```python
from build123d import *

# Parameters (mm, degrees)
CYLINDER003_R          = 4
CYLINDER003_DEPTH      = 5
CYLINDER002_R          = 4
CYLINDER002_DEPTH      = 5
CYLINDER001_R          = 4
CYLINDER001_DEPTH      = 5
CYLINDER_R             = 4
CYLINDER_DEPTH         = 5
CONE003_ROLL_ANGLE     = 90
CONE002_ROLL_ANGLE     = 90
CONE001_ROLL_ANGLE     = -90
CONE_ROLL_ANGLE        = -90
BOX001_W               = 60
BOX001_H               = 20
BOX001_DEPTH           = 50
SKETCH001_W            = 57
SKETCH001_H            = 16.7
POCKET001_DEPTH        = 50
PAD_DEPTH              = 6
BOX_W                  = 120
BOX_H                  = 20
BOX_DEPTH              = 3
SKETCH_R               = 1.75
POCKET_DEPTH           = 3.001
CHAMFER_SIZE           = 3
CHAMFER001_SIZE        = 2
FILLET_R               = 1
FILLET_PLACEMENT_ANGLE = 90


with BuildPart() as cylinder003:
    # Cylinder003 → Cylinder003 (new body)
    with BuildSketch(Plane(origin=(50, 7, 3), x_dir=(1, 0, 0), z_dir=(0, 0, 1))):
        Circle(CYLINDER003_R)
    extrude(amount=CYLINDER003_DEPTH)


with BuildPart() as cylinder002:
    # Cylinder002 → Cylinder002 (new body)
    with BuildSketch(Plane(origin=(30, 7, 3), x_dir=(1, 0, 0), z_dir=(0, 0, 1))):
        Circle(CYLINDER002_R)
    extrude(amount=CYLINDER002_DEPTH)


with BuildPart() as cylinder001:
    # Cylinder001 → Cylinder001 (new body)
    with BuildSketch(Plane(origin=(50, -7, 3), x_dir=(1, 0, 0), z_dir=(0, 0, 1))):
        Circle(CYLINDER001_R)
    extrude(amount=CYLINDER001_DEPTH)


with BuildPart() as cylinder:
    # Cylinder → Cylinder (new body)
    with BuildSketch(Plane(origin=(30, -7, 3), x_dir=(1, 0, 0), z_dir=(0, 0, 1))):
        Circle(CYLINDER_R)
    extrude(amount=CYLINDER_DEPTH)


with BuildPart() as cone003:
    # Cone003 → Cone003 (revolve)
    with BuildSketch(Plane.XZ):
        Polygon((0, 0), (3, 0), (1.75, 3), (0, 3), align=None)
    revolve(axis=Axis((0, 0, 0), (0, 0, 1)))


with BuildPart() as cone003_1:
    # Cone003 roll: moved
    add(cone003.part.rotate(Axis((0, 0, 0), (1, 0, 0)), CONE003_ROLL_ANGLE))


with BuildPart() as cone003_2:
    # Cone003 placement: moved
    add(cone003_1.part.moved(Location((75, 10, 43))))


with BuildPart() as cone002:
    # Cone002 → Cone002 (revolve)
    with BuildSketch(Plane.XZ):
        Polygon((0, 0), (3, 0), (1.75, 3), (0, 3), align=None)
    revolve(axis=Axis((0, 0, 0), (0, 0, 1)))


with BuildPart() as cone002_1:
    # Cone002 roll: moved
    add(cone002.part.rotate(Axis((0, 0, 0), (1, 0, 0)), CONE002_ROLL_ANGLE))


with BuildPart() as cone002_2:
    # Cone002 placement: moved
    add(cone002_1.part.moved(Location((105, 10, 13))))


with BuildPart() as cone001:
    # Cone001 → Cone001 (revolve)
    with BuildSketch(Plane.XZ):
        Polygon((0, 0), (3, 0), (1.75, 3), (0, 3), align=None)
    revolve(axis=Axis((0, 0, 0), (0, 0, 1)))


with BuildPart() as cone001_1:
    # Cone001 roll: moved
    add(cone001.part.rotate(Axis((0, 0, 0), (1, 0, 0)), CONE001_ROLL_ANGLE))


with BuildPart() as cone001_2:
    # Cone001 placement: moved
    add(cone001_1.part.moved(Location((105, -10, 43))))


with BuildPart() as cone:
    # Cone → Cone (revolve)
    with BuildSketch(Plane.XZ):
        Polygon((0, 0), (3, 0), (1.75, 3), (0, 3), align=None)
    revolve(axis=Axis((0, 0, 0), (0, 0, 1)))


with BuildPart() as cone_1:
    # Cone roll: moved
    add(cone.part.rotate(Axis((0, 0, 0), (1, 0, 0)), CONE_ROLL_ANGLE))


with BuildPart() as cone_2:
    # Cone placement: moved
    add(cone_1.part.moved(Location((75, -10, 13))))


with BuildPart() as obj1:
    # Box001 → Box001 (new body)
    with BuildSketch(Plane(origin=(60, -10, 3), x_dir=(1, 0, 0), z_dir=(0, 0, 1))):
        with Locations((30, 10)):
            Rectangle(BOX001_W, BOX001_H)
    extrude(amount=BOX001_DEPTH)

    # Sketch001 → Pocket001 (cut)
    with BuildSketch(Plane(origin=(60, -10, 53), x_dir=(1, 0, 0), z_dir=(0, 0, 1))):
        with Locations((31.5, 10)):
            Rectangle(SKETCH001_W, SKETCH001_H)
    extrude(amount=-POCKET001_DEPTH, mode=Mode.SUBTRACT)

    # Cut: cut Cone
    add(cone_2.part, mode=Mode.SUBTRACT)

    # Cut001: cut Cone001
    add(cone001_2.part, mode=Mode.SUBTRACT)

    # Cut002: cut Cone002
    add(cone002_2.part, mode=Mode.SUBTRACT)

    # Cut003: cut Cone003
    add(cone003_2.part, mode=Mode.SUBTRACT)


with BuildPart() as triangle:
    # Sketch002 → Pad (new body)
    with BuildSketch(Plane.XZ.offset(-3)):
        Polygon((0, 3), (60, 53), (60, 3), align=None)
    extrude(amount=PAD_DEPTH)


with BuildPart() as triangle_y:
    # Box → Box (new body)
    with BuildSketch(Plane(origin=(0, -10, 0), x_dir=(1, 0, 0), z_dir=(0, 0, 1))):
        with Locations((60, 10)):
            Rectangle(BOX_W, BOX_H)
    extrude(amount=BOX_DEPTH)

    # Sketch → Pocket (cut, through all)
    with BuildSketch(Plane(origin=(0, -10, 3), x_dir=(1, 0, 0), z_dir=(0, 0, 1))):
        with Locations((30, 17)):
            Circle(SKETCH_R)
        with Locations((30, 3)):
            Circle(SKETCH_R)
        with Locations((50, 17)):
            Circle(SKETCH_R)
        with Locations((50, 3)):
            Circle(SKETCH_R)
    extrude(amount=-POCKET_DEPTH, mode=Mode.SUBTRACT)

    # Fusion: union obj1, triangle
    add(obj1.part)
    add(triangle.part)

    # Chamfer
    chamfer_edges = [triangle_y.edges().sort_by_distance(p)[0] for p in [
        (60, -3, 28),
        (60, 3, 28),
    ]]
    chamfer(chamfer_edges, length=CHAMFER_SIZE)

    # Chamfer001
    chamfer001_edges = [triangle_y.edges().sort_by_distance(p)[0] for p in [
        (28.5, -3, 3),
        (28.5, 3, 3),
    ]]
    chamfer(chamfer001_edges, length=CHAMFER001_SIZE)

    # Cut004: cut Cylinder
    add(cylinder.part, mode=Mode.SUBTRACT)

    # Cut005: cut Cylinder001
    add(cylinder001.part, mode=Mode.SUBTRACT)

    # Cut006: cut Cylinder002
    add(cylinder002.part, mode=Mode.SUBTRACT)

    # Cut007: cut Cylinder003
    add(cylinder003.part, mode=Mode.SUBTRACT)

    # Fillet
    fillet_edges = [triangle_y.edges().sort_by_distance(p)[0] for p in [
        (0, -7.5, 3),
        (13.677124, -10, 3),
        (40, -10, 3),
        (56.322876, -10, 3),
        (60, -8, 53),
        (60, -10, 28),
        (0, 7.5, 3),
        (60, 8, 53),
        (60, 10, 28),
        (13.677124, 10, 3),
        (40, 10, 3),
        (56.322876, 10, 3),
    ]]
    fillet(fillet_edges, radius=FILLET_R)


with BuildPart() as triangle_y_1:
    # Fillet placement: moved
    add(triangle_y.part.rotate(Axis((0, 0, 0), (0, 0, 1)), FILLET_PLACEMENT_ANGLE))


solid = triangle_y_1.part
```
Source: CAD feature listing. Evaluate the final solid. Frame: model axes, mm. A direction names the side the tool comes from. Give positions to 0.01 mm unless a question says otherwise; leave off trailing zeros. Loops run counter-clockwise (first coordinate to the right, second up) from the corner with the lowest first, then second, coordinate; pieces in that order, holes last. Notation, with made-up numbers: M -11,81 L 29,81 A8 cw 29,92 Z; hole C 77,55.5 d4. An arc over 180 degrees is marked long. Put each result on its own line as item: value.
Q1. Section B-B (y = 105). Return the cut outline in (x, z).
Response values:
outline: M -10,0 L 10,0 L 10,40 L 8.35,40.69 L 8.35,3 L -8.35,3 L -8.35,10.69 L -10,10 Z; M -10,16 L -8.35,15.31 L -8.35,53 L -10,53 Z; M 8.35,45.31 L 10,46 L 10,53 L 8.35,53 Z
Q2. Line query: probe 1 along X at (y, z) = (30, 1); probe 2 along X at (y, z) = (102, 14); probe 3 along Z at (x, y) = (-5.75, 69). Output: solid intervals per line, ascending. Write a range as [from, to].
Response values:
probe 1: x = [-10, -8.75], [-5.25, 5.25], [8.75, 10]
probe 2: x = [-10, -8.35], [8.35, 10]
probe 3: z = [0, 3]
Q3. Reachability of faces 1 (the flat face through (0, 63, 28)), 2 (the flat face through (9, 85, 53)), 3 (the cylindrical face through (3, 30, 4)), 4 (the flat face through (-4, 15, 4)), 5 (the flat face through (4, 40, 4)) from +Z, -Z, +X, -X, +Y, -Y: full face, straight path, thin tool, end or side. Return the list, or none.
Response values:
face 1: +Z, +Y
face 2: +Z, +X, -X, +Y, -Y
face 3: +Z, +X
face 4: +Z, -X, -Y
face 5: +Z, +X, -Y
Q4. Section C-C (x = 1.25). Return the cut outline in (y, z).
Response values:
outline: M 0,0 L 120,0 L 120,3 L 63,3 L 63,53 L 60,53 L 0,3 Z
Q5. Pin query (flat end, axial travel): P1, Ø6, axis at x = 4.5, z = 21, coming from the +Y side; P2, Ø13.5, axis at y = 40.5, z = 19.5, coming from the +X side; P3, Ø3, axis at x = 1, z = 27.5, coming from the -Y side; P4, Ø2, axis at x = 7, y = 30, coming from the -Z side. Return the tip coordinate at first contact, or that it passes through.
Response values:
P1: stops at y = 63
P2: stops at x = 3
P3: stops at y = 27.6
P4: passes through
Q6. Section A-A (z = 13). Return the cut outline in (x, y), and give its area (3 significant figures).
Response values:
outline: M -10,61 A1 ccw -9,60 L -6,60 L -3,57 L -3,12 L 3,12 L 3,57 L 6,60 L 9,60 A1 ccw 10,61 L 10,72 L 8.35,72.69 L 8.35,63 L -8.35,63 L -8.35,102.69 L -10,102 Z; M -10,108 L -8.35,107.31 L -8.35,120 L -10,120 Z; M 8.35,77.31 L 10,78 L 10,120 L 8.35,120 Z
area: 527 mm²
Q7. Section D-D (y = 70.5). Return the cut outline in (x, z).
Response values:
outline: M -10,0 L 10,0 L 10,53 L 8.35,53 L 8.35,3 L -8.35,3 L -8.35,53 L -10,53 Z
